Could you check a few things on this model? Use its own coordinates, in mm. A direction names the side the tool comes from. Give positions to 0.01 mm unless a question says otherwise; leave off trailing zeros. Loops run counter-clockwise (first coordinate to the right, second up) from the corner with the lowest first, then second, coordinate; pieces in that order, holes last.
1. I need wall thicknesses on line 1 along Y through (x, z) = (359, 2); line 2 along X through (y, z) = (-20, 0.65). Which ranges of each line are inside material? Lowest first, please.
2. Imagine slicing it at B-B (z = 1.2). Count the separate pieces of the cut face and the enclosed holes in it, plus the area to 3 significant figures.
3. Imagine slicing it at A-A (y = -65.5). List the corners of the cut face in (x, z) for me.
4. Thinking about a two-plate mould opening in Y: for faces 3 (the flat face through (185, -85, 3)), 4 (the flat face through (6, -69.252, 3)), 5 (the flat face through (185, -42, 0)), which applies, +Y half, -Y half, draft (parallel to the pull), parting line (faces both ways), or undercut?
5. For faces 1 (the flat face through (356, -64, 3)), 2 (the flat face through (180, 0, 3)), which set-ups out of +Z, -Z, +X, -X, +Y, -Y let a thin tool reach every point of the face, with its end or its side?
```python
from build123d import *

# Parameters (mm, degrees)
SKETCH_1_R      = 1.6
SKETCH_1_W      = 6
SKETCH_1_H      = 10
SKETCH_1_W_2    = 10
SKETCH_1_H_2    = 6
EXTRUDE_1_DEPTH = 6


with BuildPart() as part:
    # Эскиз1 → Бобышка-Вытянуть1 (new body)
    with BuildSketch(Plane.XY):
        with BuildLine():
            Line((5, 0), (360, 0))
            ThreePointArc((360, 0), (363.535533906, -1.464466094), (365, -5))
            Line((365, -5), (365, -85))
            Line((365, -85), (0, -85))
            Line((0, -85), (0, -5))
            ThreePointArc((0, -5), (1.464466094, -1.464466094), (5, 0))
        make_face()
        with Locations((6, -44.251742496)):
            Circle(SKETCH_1_R, mode=Mode.SUBTRACT)
        with Locations(Location((359, -44.251742496, 0), (0, 0, 180))):
            Circle(SKETCH_1_R, mode=Mode.SUBTRACT)
        with Locations((6, -64.251742496)):
            Rectangle(SKETCH_1_W, SKETCH_1_H, mode=Mode.SUBTRACT)
        with Locations((6, -24.251742496)):
            Rectangle(SKETCH_1_W, SKETCH_1_H, mode=Mode.SUBTRACT)
        with Locations((359, -24.251742496)):
            Rectangle(SKETCH_1_W, SKETCH_1_H, mode=Mode.SUBTRACT)
        with Locations((359, -64.251742496)):
            Rectangle(SKETCH_1_W, SKETCH_1_H, mode=Mode.SUBTRACT)
        with Locations((83, -6)):
            Rectangle(SKETCH_1_W_2, SKETCH_1_H_2, mode=Mode.SUBTRACT)
        with Locations((23, -6)):
            Rectangle(SKETCH_1_W_2, SKETCH_1_H_2, mode=Mode.SUBTRACT)
        with Locations((143, -6)):
            Rectangle(SKETCH_1_W_2, SKETCH_1_H_2, mode=Mode.SUBTRACT)
        with Locations((222, -6)):
            Rectangle(SKETCH_1_W_2, SKETCH_1_H_2, mode=Mode.SUBTRACT)
        with Locations((282, -6)):
            Rectangle(SKETCH_1_W_2, SKETCH_1_H_2, mode=Mode.SUBTRACT)
        with Locations((342, -6)):
            Rectangle(SKETCH_1_W_2, SKETCH_1_H_2, mode=Mode.SUBTRACT)
    extrude(amount=EXTRUDE_1_DEPTH)


solid = part.part
```
Derived:
1. line 1: y = -85 to -69.25, -59.25 to -45.85, -42.65 to -29.25, -19.25 to 0
1. line 2: x = 0 to 3, 9 to 356, 362 to 365
2. separate pieces: 1
2. enclosed holes: 12
2. area: 30,400 mm2
3. outline: (0, 0) - (3, 0) - (3, 6) - (0, 6) - close; (9, 0) - (356, 0) - (356, 6) - (9, 6) - close; (362, 0) - (365, 0) - (365, 6) - (362, 6) - close
4. face 3: -Y half
4. face 4: undercut
4. face 5: draft
5. face 1: +Z, -Z
5. face 2: +Z, -Z, +X, -X, +Y
